from build123d import *

# Parameters (mm, degrees)
BOSS_EXTRUDE1_DEPTH     = 14
SKETCH3_R               = 2.75
CUT_EXTRUDE1_DEPTH      = 1
CUT_EXTRUDE1_DEPTH_BACK = 6
FILLET1_R               = 1
FILLET2_R               = 0.5
CHAMFER1_SIZE           = 0.25
SKETCH4_R               = 3.1
CUT_EXTRUDE2_DEPTH      = 1
SKETCH5_R               = 3.1
SKETCH5_R_2             = 3
CUT_EXTRUDE3_DEPTH      = 4
CHAMFER2_SIZE           = 0.2
CUT_EXTRUDE4_DEPTH      = 2
SKETCH7_R               = 2
BOSS_EXTRUDE2_DEPTH     = 1
SKETCH8_R               = 2
CUT_EXTRUDE5_DEPTH      = 1
SKETCH9_R               = 1.732050808
CUT_EXTRUDE6_DEPTH      = 1
CUT_EXTRUDE6_TAPER      = 45


with BuildPart() as part:
    # Sketch1 → Boss-Extrude1 (new body)
    with BuildSketch(Plane.XY):
        with BuildLine():
            Line((-21, 0), (21, 0))
            Line((21, 0), (21, 6))
            Line((21, 6), (9, 6))
            Line((9, 6), (9, 32.8))
            Line((9, 32.8), (0.5, 32.8))
            Line((0.5, 32.8), (0.5, 24.974937186))
            ThreePointArc((0.5, 24.974937186), (0, 15), (-0.5, 24.974937186))
            Line((-0.5, 24.974937186), (-0.5, 32.8))
            Line((-0.5, 32.8), (-9, 32.8))
            Line((-9, 32.8), (-9, 6))
            Line((-9, 6), (-21, 6))
            Line((-21, 6), (-21, 0))
        make_face()
    extrude(amount=BOSS_EXTRUDE1_DEPTH)

    # Sketch3 → Cut-Extrude1 (cut, two sides)
    with BuildSketch(Plane.XZ) as cut_extrude1_sk:
        with Locations((-16, 7)):
            Circle(SKETCH3_R)
        with Locations((16, 7)):
            Circle(SKETCH3_R)
    extrude(amount=CUT_EXTRUDE1_DEPTH, mode=Mode.SUBTRACT)
    extrude(cut_extrude1_sk.sketch, amount=-CUT_EXTRUDE1_DEPTH_BACK, mode=Mode.SUBTRACT)

    # Fillet1
    fillet1_edges = [part.edges().sort_by_distance(p)[0] for p in [
        (-21, 6, 7),
        (21, 6, 7),
    ]]
    fillet(fillet1_edges, radius=FILLET1_R)

    # Fillet2
    fillet2_edges = [part.edges().sort_by_distance(p)[0] for p in [
        (-9, 6, 7),
        (-9, 32.8, 7),
        (9, 32.8, 7),
        (9, 6, 7),
    ]]
    fillet(fillet2_edges, radius=FILLET2_R)

    # Chamfer1
    chamfer1_edges = [part.edges().sort_by_distance(p)[0] for p in [
        (0, 15, 0),
        (0, 15, 14),
        (13.25, 6, 7),
        (13.25, 0, 7),
        (-18.75, 6, 7),
        (-18.75, 0, 7),
    ]]
    chamfer(chamfer1_edges, length=CHAMFER1_SIZE)

    # Sketch4 → Cut-Extrude2 (cut)
    with BuildSketch(Plane.ZY.offset(9)):
        with Locations((7, 28.9)):
            Circle(SKETCH4_R)
    extrude(amount=-CUT_EXTRUDE2_DEPTH, mode=Mode.SUBTRACT)

    # Sketch5 → Cut-Extrude3 (cut)
    with BuildSketch(Plane.ZY.offset(8)):
        with Locations((7, 28.9)):
            Circle(SKETCH5_R)
        with Locations((7, 28.9)):
            Circle(SKETCH5_R_2, mode=Mode.SUBTRACT)
    extrude(amount=-CUT_EXTRUDE3_DEPTH, mode=Mode.SUBTRACT)

    # Chamfer2
    chamfer2_edges = [part.edges().sort_by_distance(p)[0] for p in [
        (-8, 28.9, 4),
    ]]
    chamfer(chamfer2_edges, length=CHAMFER2_SIZE)

    # Sketch6 → Cut-Extrude4 (cut)
    with BuildSketch(Plane.ZY.offset(8)):
        Polygon((7.225455606, 30.617314697), (5.625489649, 29.953907631), (5.400034043, 28.236592934), (6.774544394, 27.182685303), (8.374510351, 27.846092369), (8.599965957, 29.563407066), align=None)
    extrude(amount=-CUT_EXTRUDE4_DEPTH, mode=Mode.SUBTRACT)

    # Sketch7 → Boss-Extrude2 (add)
    with BuildSketch(Plane(origin=(-0.5, 0, 0), x_dir=(0, 0, -1), z_dir=(1, 0, 0))):
        with Locations((-7, 28.9)):
            Circle(SKETCH7_R)
    extrude(amount=BOSS_EXTRUDE2_DEPTH)

    # Sketch8 → Cut-Extrude5 (cut)
    with BuildSketch(Plane(origin=(9, 0, 0), x_dir=(0, 0, -1), z_dir=(1, 0, 0))):
        with Locations((-7, 28.9)):
            Circle(SKETCH8_R)
    extrude(amount=-CUT_EXTRUDE5_DEPTH, mode=Mode.SUBTRACT)

    # Sketch9 → Cut-Extrude6 (cut)
    with BuildSketch(Plane.ZY.offset(8)):
        with Locations((7, 28.9)):
            Circle(SKETCH9_R)
    extrude(amount=-CUT_EXTRUDE6_DEPTH, taper=CUT_EXTRUDE6_TAPER, mode=Mode.SUBTRACT)


solid = part.part
Check sheet for the modelled part. Datum: model origin and axes. Units: mm. A direction names the side the tool comes from. Round coordinates to 2 decimals unless told otherwise and drop trailing zeros. Order: outer loops, then holes, each group sorted by start corner. A loop starts at its lowest first (then second) coordinate and runs counter-clockwise, first axis right, second up.
(1) Scan lines: probe 1 along X at (y, z) = (27.5, 3.5); probe 2 along Z at (x, y) = (16, 4); probe 3 along X at (y, z) = (4.5, 6.75). Record each from-to range of solid material in increasing order.
(2) Cross-section at B-B, the plane y = 20. Enter the section's corners in (x, z), and give its area (3 significant figures).
(3) Cross-section at C-C, the plane y = 2.5. Enter the section's corners in (x, z).
(4) Access from +Z, -Z, +X, -X, +Y, -Y to the whole of each face (thin tool, end or side, straight path). Record for faces 3 (the flat face through (-12, 6, 7)), 4 (the cylindrical face through (8.507, 26.948, 7.434)), 5 (the conical face through (-7.88, 27.63, 6.01)).
(5) Cross-section at A-A, the plane x = 16. Enter the section's corners in (y, z).
(6) Cross-section at D-D, the plane x = 0. Enter the section's corners in (y, z).
(7) Go/stop test with flat-tipped pins: P1, Ø3.5, axis at y = 28.9, z = 7, coming from the +X side; P2, Ø3, axis at y = 16, z = 2.5, coming from the +X side; P3, Ø5, axis at x = -12.5, z = 3.5, coming from the +Y side. Record where each tip stops, or that it passes through.
(8) Draft check along Z on faces 1 (the flat face through (-7.014, 29.107, 5.514)), 2 (the cylindrical face through (-20.715, 5.699, 7.098)). Enter one of: pulls with the +Z half, pulls with the -Z half, needs draft (parallel to the pull), parting line crosses it, or undercut.
Check sheet entries:
1. probe 1: x = -9 to -0.5, 0.5 to 9
1. probe 2: z = 0 to 4.25, 9.75 to 14
1. probe 3: x = -21 to -18.74, -13.26 to 13.26, 18.74 to 21
2. outline: (-9, 0) - (-5.25, 0) - (-5, 0.25) - (-5, 13.75) - (-5.25, 14) - (-9, 14) - close; (5, 0.25) - (5.25, 0) - (9, 0) - (9, 14) - (5.25, 14) - (5, 13.75) - close
2. area: 112 mm2
3. outline: (-21, 0) - (21, 0) - (21, 14) - (-21, 14) - close; hole circle Ø5.5 at (-16, 7); hole circle Ø5.5 at (16, 7)
4. face 3: +Z, -Z, -X, +Y
4. face 4: +X
4. face 5: -X
5. outline: (0, 0) - (6, 0) - (6, 4) - (5.75, 4.25) - (0.25, 4.25) - (0, 4) - close; (0, 10) - (0.25, 9.75) - (5.75, 9.75) - (6, 10) - (6, 14) - (0, 14) - close
6. outline: (0, 0) - (14.75, 0) - (15, 0.25) - (15, 13.75) - (14.75, 14) - (0, 14) - close; circle Ø4 at (28.9, 7)
7. P1: stops at x = 8
7. P2: stops at x = 9
7. P3: stops at y = 6
8. face 1: undercut
8. face 2: needs draft
